```python
from build123d import *

# Parameters (mm, degrees)
BOSS_EXTRUDE1_DEPTH     = 12.7
SKETCH2_W               = 19.05
SKETCH2_H               = 19.05
CUT_EXTRUDE1_DEPTH      = 0.254
SKETCH3_W               = 3.175
SKETCH3_H               = 12.7
CUT_EXTRUDE2_DEPTH      = 1.27
SKETCH4_R               = 1.905
CUT_EXTRUDE3_DEPTH      = 0.254
MIRROR2_COPY_1_SKETCH_R = 1.905
MIRROR2_COPY_1_DEPTH    = 0.254
CUT_EXTRUDE4_DEPTH      = 1.016
FILLET1_R               = 3.175
F_2_56_TAPPED_HOLE1_D   = 1.778
SKETCH8_W               = 19.05
SKETCH8_H               = 8.763
CUT_EXTRUDE5_DEPTH      = 13.7
FILLET2_R               = 0.508
F_4_CLEARANCE_HOLE1_D   = 2.9464


with BuildPart() as part:
    # Sketch1 → Boss-Extrude1 (new body, symmetric)
    with BuildSketch(Plane(origin=(0, 0, 0), x_dir=(0, 0, -1), z_dir=(1, 0, 0))):
        Polygon((0, 12.7), (0, -25.908), (12.7, -25.908), (12.7, -22.733), (3.175, -22.733), (3.175, 12.7), align=None)
    extrude(amount=BOSS_EXTRUDE1_DEPTH, both=True)

    # Sketch2 → Cut-Extrude1 (cut)
    with BuildSketch(Plane.XY):
        Rectangle(SKETCH2_W, SKETCH2_H)
    extrude(amount=-CUT_EXTRUDE1_DEPTH, mode=Mode.SUBTRACT)

    # Sketch3 → Cut-Extrude2 (cut)
    with BuildSketch(Plane.XY):
        with Locations((11.1125, 0)):
            Rectangle(SKETCH3_W, SKETCH3_H)
    extrude(amount=-CUT_EXTRUDE2_DEPTH, mode=Mode.SUBTRACT)

    # Sketch4 → Cut-Extrude3 (cut)
    with BuildSketch(Plane.XY):
        with Locations((8.177961582, 8.177961582)):
            Circle(SKETCH4_R)
    cut_extrude3 = extrude(amount=-CUT_EXTRUDE3_DEPTH, mode=Mode.SUBTRACT)

    # Mirror1: Cut-Extrude3 across plane
    add(cut_extrude3.mirror(Plane(origin=(0, 0, 0), x_dir=(0, 0, 1), z_dir=(1, 0, 0))), mode=Mode.SUBTRACT)

    # Mirror2: Cut-Extrude3 across plane
    add(cut_extrude3.mirror(Plane.ZX), mode=Mode.SUBTRACT)

    # Mirror2 copy 1 sketch → Mirror2 copy 1 (cut)
    with BuildSketch(Plane(origin=(0, 0, 0), x_dir=(-1, 0, 0), z_dir=(0, 0, 1))):
        with Locations((8.177961582, 8.177961582)):
            Circle(MIRROR2_COPY_1_SKETCH_R)
    extrude(amount=-MIRROR2_COPY_1_DEPTH, mode=Mode.SUBTRACT)

    # Sketch5 → Cut-Extrude4 (cut)
    with BuildSketch(Plane.XY.offset(-0.254)):
        with BuildLine():
            Line((7.62, 4.445), (7.62, -4.445))
            ThreePointArc((7.62, -4.445), (8.177961582, -5.792038418), (9.525, -6.35))
            Line((9.525, -6.35), (9.525, 6.35))
            ThreePointArc((9.525, 6.35), (8.177961582, 5.792038418), (7.62, 4.445))
        make_face()
    extrude(amount=-CUT_EXTRUDE4_DEPTH, mode=Mode.SUBTRACT)

    # Fillet1
    fillet1_edges = [part.edges().sort_by_distance(p)[0] for p in [
        (12.7, -24.3205, -12.7),
        (-12.7, -24.3205, -12.7),
    ]]
    fillet(fillet1_edges, radius=FILLET1_R)

    # #2-56 Tapped Hole1 (through all)
    with Locations(Plane.XY):
        with Locations((-10.795, 10.795), (10.795, 10.795), (10.795, -10.795), (-10.795, -10.795)):
            Hole(F_2_56_TAPPED_HOLE1_D / 2)

    # Sketch8 → Cut-Extrude5 (cut, through all)
    with BuildSketch(Plane.XY):
        with Locations((0, -17.0815)):
            Rectangle(SKETCH8_W, SKETCH8_H)
    extrude(amount=-CUT_EXTRUDE5_DEPTH, mode=Mode.SUBTRACT)

    # Fillet2
    fillet2_edges = [part.edges().sort_by_distance(p)[0] for p in [
        (-9.525, -21.463, -1.5875),
        (-9.525, -12.7, -1.5875),
        (9.525, -12.7, -1.5875),
        (9.525, -21.463, -1.5875),
    ]]
    fillet(fillet2_edges, radius=FILLET2_R)

    # #4 Clearance Hole1 (through all)
    with Locations(Plane(origin=(0, -22.733, 0), x_dir=(1, 0, 0), z_dir=(0, 1, 0))):
        with Locations((-9.525, 9.525), (9.525, 9.525)):
            Hole(F_4_CLEARANCE_HOLE1_D / 2)


solid = part.part
```
Source: CAD feature listing. Evaluate the final solid. Frame: model axes, mm. A direction names the side the tool comes from. Coordinates: 2 decimals unless noted, no trailing zeros. Write each loop counter-clockwise with the first axis right and the second up, starting at its lowest first coordinate (ties: lowest second). Pieces come first, ordered by that corner, then holes. Notation, with made-up numbers: (9, 68.5) -> (61, 68.5) arc R34 cw to (61, 98.5) -> close; hole circle Ø6 at (3.5, 47.25). An arc over 180 degrees is marked (long way). Return JSON: item names as keys, results as strings. Group by question number.
1) Section query D-D, the plane y = 0.5. Return loops of the section in (x, z) (3 decimals).
2) Contact query for flat-ended pins moving along their axis: P1, Ø12, axis at x = -0.5, y = 9, coming from the -Z side (3 decimals); P2, Ø2.5, axis at x = -9.525, z = -9.525, coming from the +Y side; P3, Ø12, axis at x = -1, y = -13, coming from the +Z side; P4, Ø10, axis at x = 2, y = -3, coming from the +Z side. Output: stop coordinate, or through.
3) Section query A-A, the plane y = -20.5. Return loops of the section in (x, z) (3 decimals), plus the area to 3 significant figures.
4) Section query B-B, the plane x = -1.5. Return loops of the section in (y, z) (3 decimals).
5) Set-up query: faces 1 (the face through (0, -12.7, -2)), 2 (the face through (8.193, 5.807, -0.755)), 3 (the face through (0, -22.733, -8)). Return all of +Z, -Z, +X, -X, +Y, -Y with unobstructed straight access to the full face (end or side cutting, diameter ignored); none if empty.
6) Ray query, line 1 along Y through (x, z) = (10.75, -3); line 2 along Y through (x, z) = (-0.25, -1.25); line 3 along Y through (x, z) = (-4.75, -4.75). Return the intervals inside material, ascending.
7) Mould query, pull axis Z, two halves, no side actions, for faces 4 (the face through (-8.356, -24.343, -8.629)), 5 (the face through (-9.525, -17, -2)), 6 (the face through (0, -11, 0)), 7 (the face through (-11.79, -24.3, -11.75)). Classes: +Z half, -Z half, draft (parallel to the pull), parting line (faces both ways), or undercut.
8) Section query C-C, the plane z = -10.5. Return loops of the section in (x, y).
From the geometry:
{
 "1": {"outline": "(-12.7, -3.175) -> (12.7, -3.175) -> (12.7, -1.27) -> (7.62, -1.27) -> (7.62, -0.254) -> (-9.525, -0.254) -> (-9.525, 0) -> (-12.7, 0) -> close"},
 "2": {"P1": "z = -3.175", "P2": "through", "P3": "z = 0", "P4": "z = -0.25"},
 "3": {"outline": "(-12.7, -3.175) -> (-9.525, -3.175) -> (-9.525, 0) -> (-12.7, 0) -> close; (9.525, -3.175) -> (12.7, -3.175) -> (12.7, 0) -> (9.525, 0) -> close", "area": "20.2 mm²"},
 "4": {"outline": "(-25.908, -12.7) -> (-22.733, -12.7) -> (-22.733, -3.175) -> (-21.463, -3.175) -> (-21.463, 0) -> (-25.908, 0) -> close; (-12.7, -3.175) -> (12.7, -3.175) -> (12.7, 0) -> (9.525, 0) -> (9.525, -0.254) -> (-9.525, -0.254) -> (-9.525, 0) -> (-12.7, 0) -> close"},
 "5": {"face 1": "+Z, -Z", "face 2": "+Z, +X", "face 3": "-Z, +X, -X, +Y"},
 "6": {"line 1": "-25.91 to -11.68, -9.91 to 9.91, 11.68 to 12.7", "line 2": "-25.91 to -21.46, -12.7 to 12.7", "line 3": "-25.91 to -22.73"},
 "7": {"face 4": "undercut", "face 5": "draft", "face 6": "+Z half", "face 7": "-Z half"},
 "8": {"outline": "(-12.55, -25.91) -> (-10.63, -25.91) -> (-10.63, -22.73) -> (-12.55, -22.73) -> close; (-8.42, -25.91) -> (8.42, -25.91) -> (8.42, -22.73) -> (-8.42, -22.73) -> close; (10.63, -25.91) -> (12.55, -25.91) -> (12.55, -22.73) -> (10.63, -22.73) -> close"}
}
